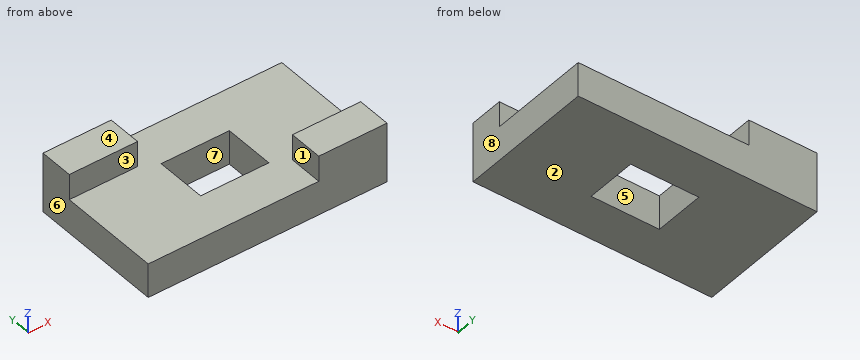
```python
from build123d import *

# Parameters (mm, degrees)
SKETCH1_W           = 56
SKETCH1_H           = 32
SKETCH1_W_2         = 16
SKETCH1_H_2         = 12
BOSS_EXTRUDE1_DEPTH = 4
SKETCH2_W           = 16
SKETCH2_H           = 8
BOSS_EXTRUDE3_DEPTH = 6


with BuildPart() as part:
    # Sketch1 → Boss-Extrude1 (new, symmetric)
    with BuildSketch(Plane.XY):
        with Locations((-28, 16)):
            Rectangle(SKETCH1_W, SKETCH1_H)
        with Locations((-28, 16)):
            Rectangle(SKETCH1_W_2, SKETCH1_H_2, mode=Mode.SUBTRACT)
    extrude(amount=BOSS_EXTRUDE1_DEPTH, both=True)

    # Sketch2 → Boss-Extrude3 (add, symmetric)
    with BuildSketch(Plane.XY.offset(4)):
        with Locations((-48, 28)):
            Rectangle(SKETCH2_W, SKETCH2_H)
        with Locations((-8, 4)):
            Rectangle(SKETCH2_W, SKETCH2_H)
    extrude(amount=BOSS_EXTRUDE3_DEPTH, both=True)


solid = part.part
```
CAD build for the part. Positions are in the model's coordinates, mm. Face numbers are marked on the shaded views. A direction names the side the tool comes from. Round coordinates to 2 decimals unless told otherwise and drop trailing zeros. Order: outer loops, then holes, each group sorted by start corner. A loop starts at its lowest first (then second) coordinate and runs counter-clockwise, first axis right, second up. Notation, with made-up numbers: (54, 16.25) -> (64, 16.25) arc R24 ccw to (64, 47.25) -> close; hole circle Ø8 at (25.5, 68). An arc over 180 degrees is marked (long way). Write item = value, one per line.
(1) Cut at C-C (z = 0.25). Write the cut outline in (x, y).
Answers follow:
outline = (-56, 0) -> (0, 0) -> (0, 32) -> (-56, 32) -> close; hole (-36, 10) -> (-20, 10) -> (-20, 22) -> (-36, 22) -> close
(2) Cut at A-A (x = -32). Write the cut outline in (y, z), plus the area to 3 significant figures.
Answers follow:
outline = (0, -4) -> (10, -4) -> (10, 4) -> (0, 4) -> close; (22, -4) -> (32, -4) -> (32, 4) -> (22, 4) -> close
area = 160 mm²
(3) Pull direction X, two halves, no side cores. Call the marked faces 6, 7 and 8: +X half, -X half, draft (parallel to the pull), parting line (faces both ways), or undercut.
Answers follow:
face_6 = -X half
face_7 = undercut
face_8 = +X half
(4) Flat gauge pins, fed straight in: P1, Ø6.5, axis at y = 28.5, z = 7.5, coming from the +X side; P2, Ø5, axis at y = 21, z = 8, coming from the +X side; P3, Ø6.5, axis at x = -6, z = 8.5, coming from the +Y side; P4, Ø3, axis at x = -48.5, z = 6, coming from the -Y side. Where does each tip first touch, or does it go through?
Answers follow:
P1 = -40
P2 = through
P3 = 8
P4 = 24
(5) 3-axis set-ups, long thin cutter, end or side, ignore diameter. For the marked faces 1, 2, 3, 4 and 5: which of +Z, -Z, +X, -X, +Y, -Y reach the whole face in a straight line?
Answers follow:
face_1 = +Z, -X, +Y, -Y
face_2 = -Z, +X, -X, +Y, -Y
face_3 = +Z, +X, -X, -Y
face_4 = +Z, +X, -X, +Y, -Y
face_5 = +Z, -Z
(6) Drill centre lines: L1, parallel to X at y = 14, z = -2.25; L2, parallel to Y at x = -23.5, z = 0.25; L3, parallel to X at y = 30.5, z = 4.25. Where is each one in solid material? Low to high.
Answers follow:
L1 = -56 to -36, -20 to 0
L2 = 0 to 10, 22 to 32
L3 = -56 to -40
(7) Cut at B-B (z = 5.25). Write the cut outline in (x, y), plus the area to 3 significant figures.
Answers follow:
outline = (-56, 24) -> (-40, 24) -> (-40, 32) -> (-56, 32) -> close; (-16, 0) -> (0, 0) -> (0, 8) -> (-16, 8) -> close
area = 256 mm²
(8) Cut at D-D (y = 25). Write the cut outline in (x, z), plus the area to 3 significant figures.
Answers follow:
outline = (-56, -4) -> (0, -4) -> (0, 4) -> (-40, 4) -> (-40, 10) -> (-56, 10) -> close
area = 544 mm²
